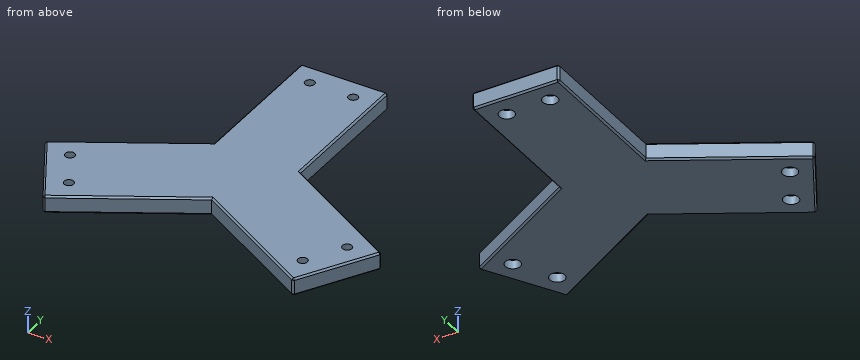
from build123d import *

# Parameters (mm, degrees)
F1_DEPTH       = 20
F2_SIZE        = 2
F4_D           = 11
F4_CBORE_D     = 17.25
F4_CBORE_DEPTH = 10


with BuildPart() as f1:
    # F0 (on Top) → F1 (new body)
    with BuildSketch(Plane.XY):
        Polygon((50, 195), (-50, 195), (-50, 28.8675134595), (-193.874953738, -54.1987298108), (-143.874953738, -140.8012701892), (0, -57.735026919), (143.874953738, -140.8012701892), (193.874953738, -54.1987298108), (50, 28.8675134595), align=None)
    extrude(amount=-F1_DEPTH)

    # F2
    f2_edges = [f1.edges().sort_by_distance(p)[0] for p in [
        (-71.937477, -99.268149, 0),
        (71.937477, -99.268149, 0),
        (168.874954, -97.5, 0),
        (121.937477, -12.665608, 0),
        (50, 111.933757, 0),
        (0, 195, 0),
        (-50, 111.933757, 0),
        (-121.937477, -12.665608, 0),
        (-168.874954, -97.5, 0),
        (-71.937477, -99.268149, -20),
        (71.937477, -99.268149, -20),
        (168.874954, -97.5, -20),
        (121.937477, -12.665608, -20),
        (50, 111.933757, -20),
        (0, 195, -20),
        (-50, 111.933757, -20),
        (-121.937477, -12.665608, -20),
        (-168.874954, -97.5, -20),
        (-143.874954, -140.80127, -10),
        (-193.874954, -54.19873, -10),
        (-50, 195, -10),
        (50, 195, -10),
        (193.874954, -54.19873, -10),
        (143.874954, -140.80127, -10),
    ]]
    chamfer(f2_edges, length=F2_SIZE)

    # F4 (through all)
    with Locations(Plane(origin=(0, 0, -20), x_dir=(1, 0, 0), z_dir=(0, 0, -1))):
        with Locations((159.7243186434, 63.3493649054), (134.7243186434, 106.6506350946), (-25, -170), (25, -170), (-134.7243186434, 106.6506350946), (-159.7243186434, 63.3493649054)):
            CounterBoreHole(F4_D / 2, F4_CBORE_D / 2, F4_CBORE_DEPTH)


with BuildPart() as f5_1:
    # F5: copy of F1
    add(f1.part)


solid = f1.part
The listing builds one solid part. Answer for the finished solid, in the listing's coordinates (mm). Coordinates: 2 decimals unless noted, no trailing zeros. Write each loop counter-clockwise with the first axis right and the second up, starting at its lowest first coordinate (ties: lowest second). Pieces come first, ordered by that corner, then holes. Notation, with made-up numbers: (27, -31.5) - (43, -31.5) arc R25 ccw to (43, -5.5) - close; hole circle Ø6 at (21.25, 54). An arc over 180 degrees is marked (long way). Put each result on its own line as item: value.
1. Find the intervals of material crossed by line 1 along X through (y, z) = (170, -16) (3 decimals); line 2 along X through (y, z) = (170, -4.75); line 3 along X through (y, z) = (-69.5, -18.5), in increasing order. Write a range as from..to.
Answer sheet:
line 1: x = -50..-33.625, -16.375..16.375, 33.625..50
line 2: x = -50..-30.5, -19.5..19.5, 30.5..50
line 3: x = -184.46..-165.77, -153.68..-21.38, 21.38..153.68, 165.77..184.46
2. The part is cut by section B-B on x = -25. Give the vertices of the cut face in (y, z) (3 decimals).
Answer sheet:
outline: (-72.169, -18) - (-69.859, -20) - (161.375, -20) - (161.375, -10) - (164.5, -10) - (164.5, 0) - (-69.859, 0) - (-72.169, -2) - close; (175.5, -10) - (178.625, -10) - (178.625, -20) - (193, -20) - (195, -18) - (195, -2) - (193, 0) - (175.5, 0) - close
3. Flat-ended cylindrical pins translate along their axes: pin 1 Ø15.5 at (x, y) = (-25, 170) entering from -Z; pin 2 Ø22.5 at (x, y) = (-159.72, -63.35) entering from -Z; pin 3 Ø5 at (y, z) = (112, -13.5) entering from +X; pin 4 Ø4 at (x, z) = (47, -16) entering from -Y. Find the tip coordinate at first contact, or state that the pin passes through.
Answer sheet:
pin 1: stops at z = -10
pin 2: stops at z = -20
pin 3: stops at x = 50
pin 4: stops at y = -86.03
4. The part is cut by section D-D on x = -68. Give the vertices of the cut face in (y, z), plus the area to 3 significant figures.
Answer sheet:
outline: (-96.99, -18) - (-94.69, -20) - (16.17, -20) - (18.48, -18) - (18.48, -2) - (16.17, 0) - (-94.69, 0) - (-96.99, -2) - close
area: 2,300 mm^2
5. The part is cut by section C-C on z = -14.5. Give the vertices of the cut face in (x, y) (3 decimals).
Answer sheet:
outline: (-192.875, -55.931) - (-144.875, -139.069) - (-142.143, -139.801) - (0, -57.735) - (142.143, -139.801) - (144.875, -139.069) - (192.875, -55.931) - (192.143, -53.199) - (50, 28.868) - (50, 193) - (48, 195) - (-48, 195) - (-50, 193) - (-50, 28.868) - (-192.143, -53.199) - close; hole circle Ø17.25 at (-159.724, -63.349); hole circle Ø17.25 at (-134.724, -106.651); hole circle Ø17.25 at (-25, 170); hole circle Ø17.25 at (25, 170); hole circle Ø17.25 at (134.724, -106.651); hole circle Ø17.25 at (159.724, -63.349)
6. The part is cut by section A-A on y = 170. Give the vertices of the cut face in (x, z) (3 decimals).
Answer sheet:
outline: (-50, -18) - (-48, -20) - (-33.625, -20) - (-33.625, -10) - (-30.5, -10) - (-30.5, 0) - (-48, 0) - (-50, -2) - close; (-19.5, -10) - (-16.375, -10) - (-16.375, -20) - (16.375, -20) - (16.375, -10) - (19.5, -10) - (19.5, 0) - (-19.5, 0) - close; (30.5, -10) - (33.625, -10) - (33.625, -20) - (48, -20) - (50, -18) - (50, -2) - (48, 0) - (30.5, 0) - close
